For this review, take the finished solid that the model builds, in its own axes (mm). Face numbers are marked on the shaded views. A direction names the side the tool comes from. Coordinates: 2 decimals unless noted, no trailing zeros. Order: outer loops, then holes, each group sorted by start corner. A loop starts at its lowest first (then second) coordinate and runs counter-clockwise, first axis right, second up. Notation, with made-up numbers: M 50.5,43 L 63.5,43 A13 cw 63.5,49 Z; hole C 30,-13.5 d2. An arc over 180 degrees is marked long. Use CSV: the item, a comma, the result in double quotes.
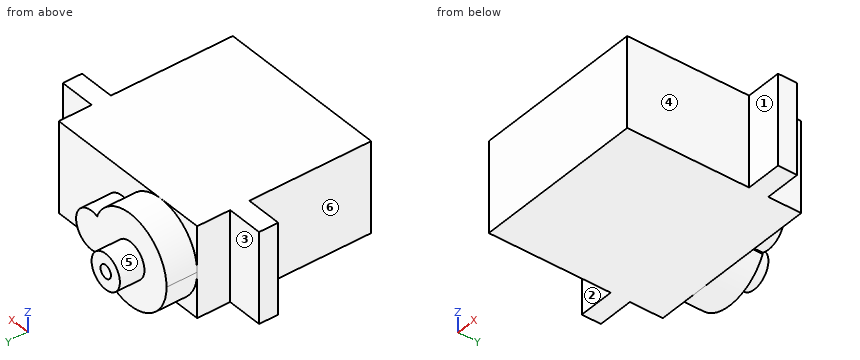
```python
from build123d import *

# Parameters (mm, degrees)
CROQUIS1_W              = 4.7
CROQUIS1_H              = 2.5
CROQUIS1_W_2            = 22.5
CROQUIS1_H_2            = 15.9
SALIENTE_EXTRUIR1_DEPTH = 11.8
SALIENTE_EXTRUIR2_DEPTH = 4
SALIENTE_EXTRUIR3_DEPTH = 3.2


with BuildPart() as part:
    # Croquis1 → Saliente-Extruir1 (new body)
    with BuildSketch(Plane.XY):
        with Locations((-13.6, 5.8)):
            Rectangle(CROQUIS1_W, CROQUIS1_H)
        Polygon((-11.25, 7.05), (-11.25, 4.55), (11.25, 4.55), (11.25, 7.05), (11.25, 11.35), (-11.25, 11.35), align=None)
        with Locations((0, -3.4)):
            Rectangle(CROQUIS1_W_2, CROQUIS1_H_2)
        with Locations((13.6, 5.8)):
            Rectangle(CROQUIS1_W, CROQUIS1_H)
    extrude(amount=SALIENTE_EXTRUIR1_DEPTH)

    # Croquis3 → Saliente-Extruir2 (add)
    with BuildSketch(Plane(origin=(0, 11.35, 0), x_dir=(1, 0, 0), z_dir=(0, 1, 0))):
        with BuildLine():
            ThreePointArc((0.066666667, -3.561256273), (0.427903311, -4.705917367), (0.55, -5.9))
            Line((0.55, -5.9), (3.45, -5.9))
            ThreePointArc((3.45, -5.9), (2.371560176, -3.84350622), (0.066666667, -3.561256273))
        make_face()
        with BuildLine():
            Line((3.45, -5.9), (0.55, -5.9))
            ThreePointArc((0.55, -5.9), (0.427903311, -7.094082633), (0.066666667, -8.238743727))
            ThreePointArc((0.066666667, -8.238743727), (2.371560176, -7.95649378), (3.45, -5.9))
        make_face()
        with BuildLine():
            Line((0, -8.212466216), (0, -5.9))
            Line((0, -5.9), (-1.55, -5.9))
            ThreePointArc((-1.55, -5.9), (-1.126655966, -7.291941091), (0, -8.212466216))
        make_face()
        with BuildLine():
            Line((-1.55, -5.9), (0, -5.9))
            Line((0, -5.9), (0, -3.587533784))
            ThreePointArc((0, -3.587533784), (-1.126655966, -4.508058909), (-1.55, -5.9))
        make_face()
        with BuildLine():
            ThreePointArc((0.066666667, -8.238743727), (0.427903311, -7.094082633), (0.55, -5.9))
            Line((0.55, -5.9), (0, -5.9))
            Line((0, -5.9), (0, -8.212466216))
            ThreePointArc((0, -8.212466216), (0.033239178, -8.225843846), (0.066666667, -8.238743727))
        make_face()
        with BuildLine():
            Line((0, -5.9), (0.55, -5.9))
            ThreePointArc((0.55, -5.9), (0.427903311, -4.705917367), (0.066666667, -3.561256273))
            ThreePointArc((0.066666667, -3.561256273), (0.033239178, -3.574156154), (0, -3.587533784))
            Line((0, -3.587533784), (0, -5.9))
        make_face()
        with BuildLine():
            ThreePointArc((0, -8.212466216), (-1.126655966, -7.291941091), (-1.55, -5.9))
            Line((-1.55, -5.9), (-11.25, -5.9))
            ThreePointArc((-11.25, -5.9), (-6.62377392, -11.660859311), (0, -8.387468593))
            Line((0, -8.387468593), (0, -8.212466216))
        make_face()
        with BuildLine():
            Line((-11.25, -5.9), (-1.55, -5.9))
            ThreePointArc((-1.55, -5.9), (-1.126655966, -4.508058909), (0, -3.587533784))
            Line((0, -3.587533784), (0, -3.412531407))
            ThreePointArc((0, -3.412531407), (-6.62377392, -0.139140689), (-11.25, -5.9))
        make_face()
    extrude(amount=SALIENTE_EXTRUIR2_DEPTH)

    # Croquis4 → Saliente-Extruir3 (add)
    with BuildSketch(Plane(origin=(0, 15.35, 0), x_dir=(1, 0, 0), z_dir=(0, 1, 0))):
        with BuildLine():
            ThreePointArc((-6.2, -5.9), (-5.35, -5.05), (-4.5, -5.9))
            Line((-4.5, -5.9), (-3.05, -5.9))
            ThreePointArc((-3.05, -5.9), (-5.35, -3.6), (-7.65, -5.9))
            Line((-7.65, -5.9), (-6.2, -5.9))
        make_face()
        with BuildLine():
            Line((-3.05, -5.9), (-4.5, -5.9))
            ThreePointArc((-4.5, -5.9), (-5.35, -6.75), (-6.2, -5.9))
            Line((-6.2, -5.9), (-7.65, -5.9))
            ThreePointArc((-7.65, -5.9), (-5.35, -8.2), (-3.05, -5.9))
        make_face()
    extrude(amount=SALIENTE_EXTRUIR3_DEPTH)


solid = part.part
```
Item 1: To check wall thickness, follow line 1 along Z through (x, y) = (-5.35, 16.3); line 2 along Y through (x, z) = (-14, 3); line 3 along Y through (x, z) = (3, 1). State the ranges of each line that lie inside material, in increasing order. Write a range as [from, to].
Solutions:
line 1,"[3.6, 5.05], [6.75, 8.2]"
line 2,"[4.55, 7.05]"
line 3,"[-11.35, 11.35]"
Item 2: Add section B-B on x = 0.5. State the section outline as (y, z) points.
Solutions:
outline,"M -11.35,0 L 11.35,0 L 11.35,3.44 L 15.35,3.44 L 15.35,8.36 L 11.35,8.36 L 11.35,11.8 L -11.35,11.8 Z"
Item 3: Clearance check with flat-ended pins moving along their axes: pin 1 Ø1.4 at (x, z) = (-14.5, 8) entering from +Y; pin 2 Ø1 at (y, z) = (14.5, 5.5) entering from +X; pin 3 Ø2 at (y, z) = (9, 8.5) entering from -X. State where each tip first meets the part, or that it passes through.
Solutions:
pin 1,"y = 7.05"
pin 2,"x = 3.45"
pin 3,"x = -11.25"
Item 4: Add section D-D on y = 2. State the section outline as (x, z) points.
Solutions:
outline,"M -11.25,0 L 11.25,0 L 11.25,11.8 L -11.25,11.8 Z"
Item 5: For the marked faces 1, 2 and 3, list the 3-axis set-ups (+Z, -Z, +X, -X, +Y, -Y) from which the entire face can be reached by the end or side of a thin tool; tool diameter is ignored.
Solutions:
face 1,"+Z, -Z, +X, -Y"
face 2,"+Z, -Z, -X, -Y"
face 3,"+Z, -Z, -X, +Y"
Item 6: Add section A-A on y = 16.5. State the section outline as (x, z) points, and give its area (3 significant figures).
Solutions:
outline,"C -5.35,5.9 d4.6; hole C -5.35,5.9 d1.7"
area,"14.3 mm^2"
Item 7: Add section C-C on z = 4. State the section outline as (x, y) points.
Solutions:
outline,"M -15.95,4.55 L -11.25,4.55 L -11.25,-11.35 L 11.25,-11.35 L 11.25,4.55 L 15.95,4.55 L 15.95,7.05 L 11.25,7.05 L 11.25,11.35 L 2.57,11.35 L 2.57,15.35 L -4.05,15.35 L -4.05,18.55 L -6.65,18.55 L -6.65,15.35 L -10.94,15.35 L -10.94,11.35 L -11.25,11.35 L -11.25,7.05 L -15.95,7.05 Z"
Item 8: Draft analysis for pull direction X (two halves, no side actions). For the marked faces 4, 5 and 6, state which applies: released by +X, released by -X, zero draft, split by the parting line, or undercut.
Solutions:
face 4,"released by +X"
face 5,"split by the parting line"
face 6,"released by -X"
